from build123d import *

# Parameters (mm, degrees)
F1_DEPTH = 3.81
F2_W     = 34.925
F2_H     = 3.81
F3_DEPTH = 6.35
F4_W     = 34.925
F4_H     = 3.175
F5_DEPTH = 2.54
F6_R     = 1.5875


with BuildPart() as f1:
    # F0 (on Right) → F1 (new body)
    with BuildSketch(Plane.YZ):
        with BuildLine():
            Line((0, 34.925), (0, 0))
            Line((0, 0), (34.925, 0))
            Line((34.925, 0), (34.925, 15.875))
            ThreePointArc((34.925, 15.875), (33.995064, 18.120064), (31.75, 19.05))
            Line((31.75, 19.05), (15.875, 19.05))
            ThreePointArc((15.875, 19.05), (11.384872, 20.909872), (9.525, 25.4))
            Line((9.525, 25.4), (9.525, 34.925))
            ThreePointArc((9.525, 34.925), (8.595064, 37.170064), (6.35, 38.1))
            Line((6.35, 38.1), (3.175, 38.1))
            ThreePointArc((3.175, 38.1), (0.929936, 37.170064), (0, 34.925))
        make_face()
    extrude(amount=F1_DEPTH)

    # F2 (on face) → F3 (join)
    with BuildSketch(Plane.YZ.offset(3.81)):
        with Locations((17.4625, 1.905)):
            Rectangle(F2_W, F2_H)
    extrude(amount=F3_DEPTH)

    # F4 (on face) → F5 (join)
    with BuildSketch(Plane(origin=(0, 0, 0), x_dir=(0, -1, 0), z_dir=(-1, 0, 0))):
        with Locations((-17.4625, 1.5875)):
            Rectangle(F4_W, F4_H)
    extrude(amount=F5_DEPTH)

    # F6
    f6_edges = [f1.edges().sort_by_distance(p)[0] for p in [
        (3.81, 17.4625, 3.81),
        (10.16, 17.4625, 3.81),
        (0, 17.4625, 3.175),
        (10.16, 17.4625, 0),
    ]]
    fillet(f6_edges, radius=F6_R)

    # F7: F1 across face


with BuildPart() as f1_1:
    add(f1.part)
    add(f1.part.mirror(Plane(origin=(-2.54, 17.4625, 1.5875), x_dir=(0, -1, 0), z_dir=(-1, 0, 0))))


solid = f1_1.part
Verification items for the finished model (mm, model axes). A direction names the side the tool comes from. Give positions to 0.01 mm unless a question says otherwise; leave off trailing zeros. Write each loop counter-clockwise with the first axis right and the second up, starting at its lowest first coordinate (ties: lowest second). Pieces come first, ordered by that corner, then holes. Notation, with made-up numbers: (-9.75, 63.25) - (47.25, 63.25) arc R20 cw to (47.25, 94.25) - close; hole circle Ø8 at (28, -32). An arc over 180 degrees is marked (long way). Answer as CSV lines item,"result". Start each with the question number.
1. Depth check by flat-ended pin: pin 1 (10 mm diameter, centred on x = 5, z = 23, fed in from +Y); pin 2 (4 mm diameter, centred on x = 2.5, y = 22.5, fed in from +Z); pin 3 (1.9 mm diameter, centred on x = 2.5, z = 32.5, fed in from +Y) (3 decimals); pin 4 (4 mm diameter, centred on x = 2.5, y = 7, fed in from +Z). Enter the tip coordinate at first touch or a pass-through.
2. Draft check along X on faces 4 (the face through (3.81, 13, 18)), 5 (the face through (-6.958, 11.435, 20.861)), 6 (the face through (-3, 18, 3.175)), 7 (the face through (-14.76, 17.71, 0.45)). Enter one of: pulls with the +X half, pulls with the -X half, needs draft (parallel to the pull), parting line crosses it, or undercut.
3. Set-up check for faces 1 (the face through (7, 17, 3.81)), 2 (the face through (2, 5, 38.1)), 3 (the face through (2, 9.525, 30)): record each of +Z, -Z, +X, -X, +Y, -Y from which the full face is reachable in a straight line by a thin tool's end or side.
4. Sectioned sample at D-D (z = 21). Record the boundary of the cut face in (x, y).
5. Thickness scan on line 1 (X direction, y = 7, z = 20); line 2 (Z direction, x = 5.5, y = 33); line 3 (Z direction, x = -3, y = 9) (3 decimals). Record the ranges inside material, lowest first.
6. Sectioned sample at C-C (x = -8). Record the boundary of the cut face in (y, z) (3 decimals), then the cut area to 3 significant figures.
7. Sectioned sample at A-A (z = 10). Record the boundary of the cut face in (x, y) (3 decimals).
Derived:
1,pin 1,"y = 33.97"
1,pin 2,"z = 19.05"
1,pin 3,"y = 9.525"
1,pin 4,"z = 38.1"
2,face 4,"pulls with the +X half"
2,face 5,"needs draft"
2,face 6,"undercut"
2,face 7,"pulls with the -X half"
3,face 1,"+Z, +X, +Y, -Y"
3,face 2,"+Z, +X, -X, +Y, -Y"
3,face 3,"+Z, +X, -X, +Y"
4,outline,"(-8.89, 0) - (-5.08, 0) - (-5.08, 11.3) - (-8.89, 11.3) - close; (0, 0) - (3.81, 0) - (3.81, 11.3) - (0, 11.3) - close"
5,line 1,"-8.89 to -5.08, 0 to 3.81"
5,line 2,"0 to 3.81"
5,line 3,"0 to 3.175"
6,outline,"(0, 0) - (34.925, 0) - (34.925, 15.875) arc R3.175 ccw to (31.75, 19.05) - (15.875, 19.05) arc R6.35 cw to (9.525, 25.4) - (9.525, 34.925) arc R3.175 ccw to (6.35, 38.1) - (3.175, 38.1) arc R3.175 ccw to (0, 34.925) - close"
6,area,"849 mm²"
7,outline,"(-8.89, 0) - (-5.08, 0) - (-5.08, 34.925) - (-8.89, 34.925) - close; (0, 0) - (3.81, 0) - (3.81, 34.925) - (0, 34.925) - close"
